Part model, mm, in its own coordinate system. A direction names the side the tool comes from. Round coordinates to 2 decimals unless told otherwise and drop trailing zeros. Write each loop counter-clockwise with the first axis right and the second up, starting at its lowest first coordinate (ties: lowest second). Pieces come first, ordered by that corner, then holes. Notation, with made-up numbers: (63, 32.25) -> (71, 32.25) arc R36 cw to (71, 70.25) -> close; hole circle Ø10 at (-40, 36). An arc over 180 degrees is marked (long way). Return JSON: item names as keys, results as strings. Group by question number.
(1) Tool access for faces 4 (the flat face through (29, 3, 93.7)), 5 (the flat face through (-2, 0, 5)): list every direction of +Z, -Z, +X, -X, +Y, -Y with a clear straight run to the whole face (end or side of a thin tool).
(2) Drop flat-ended pins along their axis: pin 1 Ø0.9 at (y, z) = (3.5, 92.5) entering from -X; pin 2 Ø2 at (y, z) = (5.5, -19.5) entering from +X; pin 3 Ø1 at (y, z) = (0.5, 17) entering from +X. Give the stop position or say it passes through.
(3) Saw through at B-B (z = -22.5). List the corners of the cut face in (x, y).
(4) Saw through at A-A (y = 2). State how many separate pieces and enclosed holes the cut face has, plus the area to 3 significant figures.
(5) Saw through at D-D (z = 33.5). List the corners of the cut face in (x, y).
(6) Saw through at C-C (x = -78). List the corners of the cut face in (y, z), plus the area to 3 significant figures.
(7) Drill centre lines: L1, parallel to X at y = 4.75, z = -18.5; L2, parallel to Z at x = -28, y = 5.25; L3, parallel to X at y = 0.5, z = -70. Where is each one in solid material? Low to high. Write a range as from..to.
(8) Mould opens along X. For faces 1 (the flat face through (86.906, 3.131, -49.475)), 2 (the flat face through (-95.584, 3.219, -21.844)), 3 (the flat face through (-76.232, 3.131, 42.963)) say: +X half, -X half, draft (parallel to the pull), parting line (faces both ways), or undercut.
from build123d import *

# Parameters (mm, degrees)
BOSS_EXTRUDE1_DEPTH = 6.35
SKETCH2_W           = 18
SKETCH2_H           = 3
CUT_EXTRUDE1_DEPTH  = 148.509567486


with BuildPart() as part:
    # Sketch1 → Boss-Extrude1 (new body)
    with BuildSketch(Plane(origin=(0, 0, 0), x_dir=(1, 0, 0), z_dir=(0, 1, 0))):
        Polygon((64.951905284, 87.5), (-64.951905284, 87.5), (-108.253175473, 12.5), (-43.301270189, -100), (43.301270189, -100), (108.253175473, 12.5), align=None)
    extrude(amount=BOSS_EXTRUDE1_DEPTH)

    # Sketch2 → Cut-Extrude1 (cut, through all)
    with BuildSketch(Plane(origin=(0, 6.35, 0), x_dir=(1, 0, 0), z_dir=(0, 1, 0))):
        with Locations((-29, -92.2)):
            Rectangle(SKETCH2_W, SKETCH2_H)
        with Locations((29, -92.2)):
            Rectangle(SKETCH2_W, SKETCH2_H)
        Polygon((-62.146580335, 79.758965344), (-59.548504123, 78.258965344), (-68.548504123, 62.670508076), (-71.146580335, 64.170508076), align=None)
        Polygon((-97.548504123, 12.441034656), (-88.548504123, 28.029491924), (-91.146580335, 29.529491924), (-100.146580335, 13.941034656), align=None)
        Polygon((100.146580335, 13.941034656), (91.146580335, 29.529491924), (88.548504123, 28.029491924), (97.548504123, 12.441034656), align=None)
        Polygon((59.548504123, 78.258965344), (62.146580335, 79.758965344), (71.146580335, 64.170508076), (68.548504123, 62.670508076), align=None)
    extrude(amount=-CUT_EXTRUDE1_DEPTH, mode=Mode.SUBTRACT)


solid = part.part
Computed values:
{
 "1": {"face 4": "+Y, -Y", "face 5": "+Z, -Z, +X, -X, -Y"},
 "2": {"pin 1": "x = -47.89", "pin 2": "x = 104.79", "pin 3": "x = 91.51"},
 "3": {"outline": "(-102.48, 0) -> (-95.21, 0) -> (-95.21, 6.35) -> (-102.48, 6.35) -> close; (-91.74, 0) -> (91.74, 0) -> (91.74, 6.35) -> (-91.74, 6.35) -> close; (95.21, 0) -> (102.48, 0) -> (102.48, 6.35) -> (95.21, 6.35) -> close"},
 "4": {"separate pieces": "1", "enclosed holes": "6", "area": "29,700 mm2"},
 "5": {"outline": "(-81.7, 0) -> (81.7, 0) -> (81.7, 6.35) -> (-81.7, 6.35) -> close"},
 "6": {"outline": "(0, -64.9) -> (6.35, -64.9) -> (6.35, 39.9) -> (0, 39.9) -> close", "area": "665 mm2"},
 "7": {"L1": "-104.79..-97.51, -94.05..94.05, 97.51..104.79", "L2": "-87.5..90.7, 93.7..100", "L3": "-75.06..-67.78, -64.32..64.32, 67.78..75.06"},
 "8": {"face 1": "+X half", "face 2": "undercut", "face 3": "-X half"}
}
